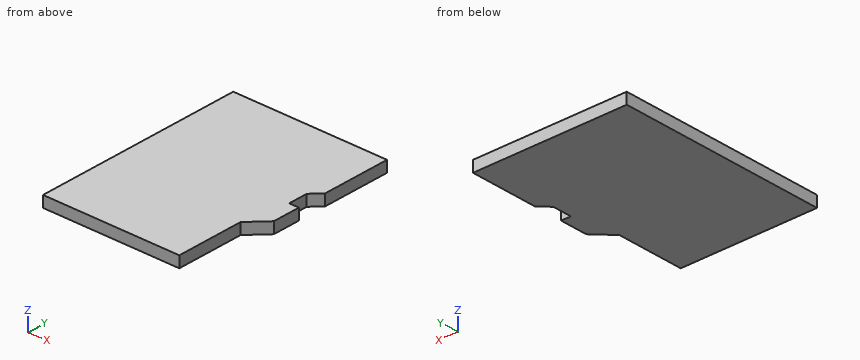
from build123d import *

# Parameters (mm, degrees)
CROQUIS1_W              = 9.84
CROQUIS1_H              = 4.9
SALIENTE_EXTRUIR1_DEPTH = 0.8


with BuildPart() as part:
    # Croquis1 → Saliente-Extruir1 (new body)
    with BuildSketch(Plane.XY):
        Polygon((-5.55, -2.7), (4.29, -2.7), (5.55, -1.44), (5.55, 0.56), (4.85, 0.56), (4.85, 1.96), (5.55, 2.66), (5.55, 7.6), (-5.55, 7.6), align=None)
        with Locations((-0.63, -5.15)):
            Rectangle(CROQUIS1_W, CROQUIS1_H)
    extrude(amount=SALIENTE_EXTRUIR1_DEPTH)


solid = part.part
Can you work these out from the model? Positions are in its coordinate system, mm. Give positions to 0.01 mm unless a question says otherwise; leave off trailing zeros. Loops run counter-clockwise (first coordinate to the right, second up) from the corner with the lowest first, then second, coordinate; pieces in that order, holes last. Notation, with made-up numbers: (27.5, 26.25) -> (64.5, 26.25) arc R7 cw to (64.5, 37.25) -> close; hole circle Ø7 at (2, 76.5). An arc over 180 degrees is marked (long way). Use one line per item in the form item = value.
1) If we section it at B-B (y = 1.5): Please give me the cut outline in (x, z), plus the area to 3 significant figures.
Answers:
outline = (-5.55, 0) -> (4.85, 0) -> (4.85, 0.8) -> (-5.55, 0.8) -> close
area = 8.32 mm²
2) I need wall thicknesses on line 1 along X through (y, z) = (1.5, 0.35); line 2 along X through (y, z) = (-6.75, 0.2). Which ranges of each line are inside material? Lowest first, please.
Answers:
line_1 = -5.55 to 4.85
line_2 = -5.55 to 4.29
3) If we section it at A-A (z = 0.35): Please give me the cut outline in (x, y), plus the area to 3 significant figures.
Answers:
outline = (-5.55, -7.6) -> (4.29, -7.6) -> (4.29, -2.7) -> (5.55, -1.44) -> (5.55, 0.56) -> (4.85, 0.56) -> (4.85, 1.96) -> (5.55, 2.66) -> (5.55, 7.6) -> (-5.55, 7.6) -> close
area = 161 mm²
4) If we section it at C-C (y = -2.25): Please give me the cut outline in (x, z), plus the area to 3 significant figures.
Answers:
outline = (-5.55, 0) -> (4.74, 0) -> (4.74, 0.8) -> (-5.55, 0.8) -> close
area = 8.23 mm²
